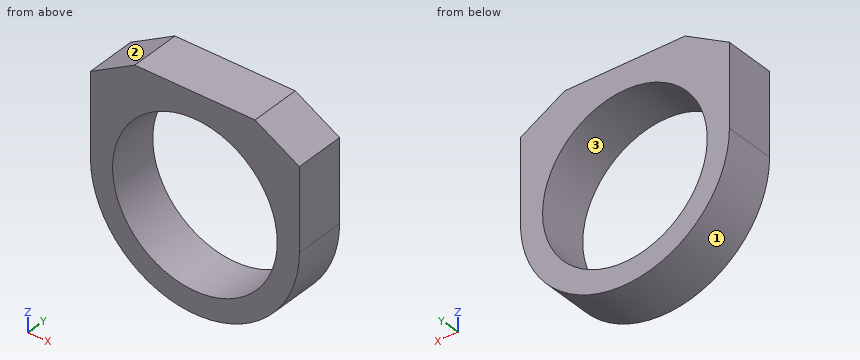
from build123d import *

# Parameters (mm, degrees)
F0_R     = 8.255
F1_DEPTH = 5.08


with BuildPart() as f1:
    # F0 (on Front) → F1 (new body)
    with BuildSketch(Plane.XZ):
        with BuildLine():
            ThreePointArc((-10.4775, 0), (0, 10.4775), (10.4775, 0))
            Line((10.4775, 0), (10.4775, 8.255))
            Line((10.4775, 8.255), (6.0325, 10.795))
            Line((6.0325, 10.795), (-6.0325, 10.795))
            Line((-6.0325, 10.795), (-10.4775, 8.255))
            Line((-10.4775, 8.255), (-10.4775, 0))
        make_face()
        with BuildLine():
            ThreePointArc((-10.4775, 0), (0, -10.4775), (10.4775, 0))
            ThreePointArc((10.4775, 0), (0, 10.4775), (-10.4775, 0))
        make_face()
        Circle(F0_R, mode=Mode.SUBTRACT)
    extrude(amount=F1_DEPTH)


solid = f1.part
Could you check a few things on this model? Use its own coordinates, in mm. Face numbers are marked on the shaded views. Coordinates: 2 decimals unless noted, no trailing zeros. Loops run counter-clockwise (first coordinate to the right, second up) from the corner with the lowest first, then second, coordinate; pieces in that order, holes last.
1. I need wall thicknesses on L1, parallel to Z at x = 0, y = -1.9 (1 decimal); L2, parallel to X at y = -1.15, z = -0.5; L3, parallel to X at y = -2.75, z = 1.75. Which ranges of each line are inside material? Lowest first, please.
2. Imagine slicing it at C-C (z = -5.5). Please give me the cut outline in (x, y).
3. For P1, Ø3, axis at y = -0.5, z = -3.5, coming from the +X side; P2, Ø3, axis at y = -2, z = -0.5, coming from the -X side, each with a flat end and sliding along its axis, tell me the tip position at first contact or that it passes through.
4. Imagine slicing it at B-B (y = -2.9). Please give me the cut outline in (x, z) (1 decimal).
5. Imagine slicing it at A-A (x = 0). Please give me the cut outline in (y, z) (1 decimal), and give its area (3 significant figures).
6. Imagine slicing it at D-D (z = 8.5). Please give me the cut outline in (x, y), and give its area (3 significant figures).
7. We'd pull the mould along Z, two halves only. Please class the marked faces 1, 2 and 3: released by +Z, released by -Z, zero draft, split by the parting line, or undercut.
Computed values:
1. L1: z = -10.5 to -8.3, 8.3 to 10.8
1. L2: x = -10.47 to -8.24, 8.24 to 10.47
1. L3: x = -10.48 to -8.07, 8.07 to 10.48
2. outline: (-8.92, -5.08) - (-6.16, -5.08) - (-6.16, 0) - (-8.92, 0) - close; (6.16, -5.08) - (8.92, -5.08) - (8.92, 0) - (6.16, 0) - close
3. P1: stops at x = 10.28
3. P2: stops at x = -10.48
4. outline: (-10.5, 0) arc R10.5 ccw to (10.5, 0) - (10.5, 8.3) - (6, 10.8) - (-6, 10.8) - (-10.5, 8.3) - close; hole circle Ø16.5 at (0, 0)
5. outline: (-5.1, -10.5) - (0, -10.5) - (0, -8.3) - (-5.1, -8.3) - close; (-5.1, 8.3) - (0, 8.3) - (0, 10.8) - (-5.1, 10.8) - close
5. area: 24.2 mm2
6. outline: (-10.05, -5.08) - (10.05, -5.08) - (10.05, 0) - (-10.05, 0) - close
6. area: 102 mm2
7. face 1: released by -Z
7. face 2: released by +Z
7. face 3: undercut
